```python
from build123d import *

# Parameters (mm, degrees)
F2_R = 8.89
F4_R = 5.08


# Not quite as in the source:
# - a fillet or chamfer that OpenCascade refuses, or shapes differently, is made with other operations: its cross-section is extruded or revolved along the edge and cut away or added


with BuildPart() as f1:
    # F0 (on Front) → F1 (revolve)
    with BuildSketch(Plane.XZ):
        Polygon((-19.955041249, 4.445), (-19.955041249, 0), (43.544958751, 0), (43.544958751, 8.89), (-12.335041249, 8.89), (-12.335041249, 4.445), align=None)
    revolve(axis=Axis((11.794958751, 0, 0), (1, 0, 0)))

    # F2
    f2_edges = [f1.edges().sort_by_distance(p)[0] for p in [
        (43.544959, 0, -8.89),
    ]]
    fillet(f2_edges, radius=F2_R)

    # F3: fillet of radius 7.62 on 1 edges, made by hand

    # F3_s1 → F3_t2 (revolve, cut)
    with BuildSketch(Plane.XZ):
        with BuildLine():
            ThreePointArc((-5.4080090562, 8.89), (-9.5232793997, 7.6831856359), (-12.335041249, 4.445))
            Line((-12.335041249, 4.445), (-12.335041249, 8.89))
            Line((-12.335041249, 8.89), (-5.4080090562, 8.89))
        make_face()
    revolve(axis=Axis((-12.335041249, 0, 0), (1, 0, 0)), mode=Mode.SUBTRACT)

    # F4
    f4_edges = [f1.edges().sort_by_distance(p)[0] for p in [
        (-12.335041, 0, -4.445),
    ]]
    fillet(f4_edges, radius=F4_R)

    # F5: chamfer of 0.635 x 1.0998522628 on 1 edges, made by hand

    # F5_s1 → F5_t2 (revolve, cut)
    with BuildSketch(Plane.XZ):
        Polygon((-18.8551889862, 4.445), (-19.955041249, 3.81), (-19.955041249, 4.445), align=None)
    revolve(axis=Axis((-19.955041249, 0, 0), (1, 0, 0)), mode=Mode.SUBTRACT)


solid = f1.part
```
Build history of the part. All positions in model axes, mm. A direction names the side the tool comes from. Give positions to 0.01 mm unless a question says otherwise; leave off trailing zeros. Loops run counter-clockwise (first coordinate to the right, second up) from the corner with the lowest first, then second, coordinate; pieces in that order, holes last. Notation, with made-up numbers: (-21, -9.75) -> (13, -9.75) arc R24 cw to (13, 11.25) -> close; hole circle Ø3 at (56.25, -25.75). An arc over 180 degrees is marked (long way). One line per question, with ' | ' between items. Start each with the question number.
1) Probe L1, parallel to X at y = 1.5, z = -2; L2, parallel to Y at x = 33, z = 5.5; L3, parallel to X at y = -0.25, z = 4.25. List the from-to ranges inside material, lowest first.
2) Pin check, flat tips, straight feed: pin 1 (8 mm diameter, centred on x = 12.5, z = 6, fed in from +Y); pin 2 (1.5 mm diameter, centred on y = -5.5, z = 6.5, fed in from +X); pin 3 (8 mm diameter, centred on y = 7, z = 5.5, fed in from -X). Stop position of each tip, or through.
3) 3-axis set-ups, long thin cutter, end or side, ignore diameter. For faces 1 (the cylindrical face through (-16.98, 2.7, -3.53)), 2 (the flat face through (-19.955, 0, 0)): which of +Z, -Z, +X, -X, +Y, -Y reach the whole face in a straight line?
4) Cut at A-A (x = 13). Give the cut face in (y, z).
Return value:
1) L1: -19.96 to 43.19 | L2: -6.98 to 6.98 | L3: -19.18 to 42.46
2) pin 1: y = 8.66 | pin 2: x = 38.98 | pin 3: x = -12.95
3) face 1: -X | face 2: +Z, -Z, -X, +Y, -Y
4) outline: circle Ø17.78 at (0, 0)
